Can you work these out from the model? Positions are in its coordinate system, mm. Give positions to 0.01 mm unless a question says otherwise; leave off trailing zeros. Order: outer loops, then holes, each group sorted by start corner. A loop starts at its lowest first (then second) coordinate and runs counter-clockwise, first axis right, second up. Notation, with made-up numbers: M 63,11.5 L 101,11.5 A15 ccw 101,39.5 Z; hole C 82.5,-18 d1. An arc over 180 degrees is marked long. Use one line per item in the form item = value. Start each with the question number.
1. I need wall thicknesses on L1, parallel to X at y = -109, z = 0.95; L2, parallel to Y at x = 61.5, z = 1.2; L3, parallel to Y at x = 182, z = 0.8. Which ranges of each line are inside material? Lowest first, please.
2. I want a section at B-B, the plane x = 152.5. List the corners of the cut face in (y, z) for me.
3. Will these pins go through, and if not, where does the flat tip stop? P1, Ø0.5, axis at x = 234, z = 1.5, coming from the -Y side; P2, Ø0.5, axis at y = -172, z = 1.5, coming from the +X side; P3, Ø0.8, axis at y = -52.5, z = 1.5, coming from the -X side.
4. I want a section at C-C, the plane y = -97. List the corners of the cut face in (x, z) for me, and give its area (3 significant figures).
5. I want a section at A-A, the plane z = 1.55. Count the separate pieces of the cut face and the enclosed holes in it, and give its area (3 significant figures).
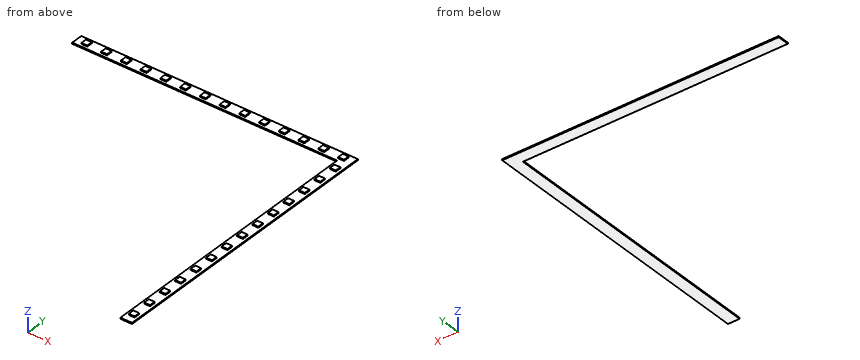
```python
from build123d import *

# Parameters (mm, degrees)
EXTRUDE_1_DEPTH = 1
SKETCH_2_W      = 5
SKETCH_2_H      = 5
EXTRUDE_2_DEPTH = 1


with BuildPart() as part:
    # 草圖1 → 填料-伸長1 (new body)
    with BuildSketch(Plane.XY):
        Polygon((0, 0), (238, 0), (238, -10), (238, -248), (228, -248), (228, -10), (0, -10), align=None)
    extrude(amount=EXTRUDE_1_DEPTH)

    # 草圖2 → 填料-伸長2 (add)
    with BuildSketch(Plane.XY.offset(1)):
        with Locations((25.5, -5)):
            Rectangle(SKETCH_2_W, SKETCH_2_H)
        with Locations((8.5, -5)):
            Rectangle(SKETCH_2_W, SKETCH_2_H)
        with Locations((42.5, -5)):
            Rectangle(SKETCH_2_W, SKETCH_2_H)
        with Locations((59.5, -5)):
            Rectangle(SKETCH_2_W, SKETCH_2_H)
        with Locations((76.5, -5)):
            Rectangle(SKETCH_2_W, SKETCH_2_H)
        with Locations((93.5, -5)):
            Rectangle(SKETCH_2_W, SKETCH_2_H)
        with Locations((110.5, -5)):
            Rectangle(SKETCH_2_W, SKETCH_2_H)
        with Locations((127.5, -5)):
            Rectangle(SKETCH_2_W, SKETCH_2_H)
        with Locations((144.5, -5)):
            Rectangle(SKETCH_2_W, SKETCH_2_H)
        with Locations((161.5, -5)):
            Rectangle(SKETCH_2_W, SKETCH_2_H)
        with Locations((178.5, -5)):
            Rectangle(SKETCH_2_W, SKETCH_2_H)
        with Locations((195.5, -5)):
            Rectangle(SKETCH_2_W, SKETCH_2_H)
        with Locations((212.5, -5)):
            Rectangle(SKETCH_2_W, SKETCH_2_H)
        with Locations((229.5, -5)):
            Rectangle(SKETCH_2_W, SKETCH_2_H)
        with Locations((233, -222.5)):
            Rectangle(SKETCH_2_W, SKETCH_2_H)
        with Locations((233, -239.5)):
            Rectangle(SKETCH_2_W, SKETCH_2_H)
        with Locations((233, -205.5)):
            Rectangle(SKETCH_2_W, SKETCH_2_H)
        with Locations((233, -188.5)):
            Rectangle(SKETCH_2_W, SKETCH_2_H)
        with Locations((233, -171.5)):
            Rectangle(SKETCH_2_W, SKETCH_2_H)
        with Locations((233, -154.5)):
            Rectangle(SKETCH_2_W, SKETCH_2_H)
        with Locations((233, -137.5)):
            Rectangle(SKETCH_2_W, SKETCH_2_H)
        with Locations((233, -120.5)):
            Rectangle(SKETCH_2_W, SKETCH_2_H)
        with Locations((233, -103.5)):
            Rectangle(SKETCH_2_W, SKETCH_2_H)
        with Locations((233, -86.5)):
            Rectangle(SKETCH_2_W, SKETCH_2_H)
        with Locations((233, -69.5)):
            Rectangle(SKETCH_2_W, SKETCH_2_H)
        with Locations((233, -52.5)):
            Rectangle(SKETCH_2_W, SKETCH_2_H)
        with Locations((233, -35.5)):
            Rectangle(SKETCH_2_W, SKETCH_2_H)
        with Locations((233, -18.5)):
            Rectangle(SKETCH_2_W, SKETCH_2_H)
    extrude(amount=EXTRUDE_2_DEPTH)


solid = part.part
```
Check result:
q1.L1 = 228 to 238
q1.L2 = -7.5 to -2.5
q1.L3 = -10 to 0
q2.outline = M -10,0 L 0,0 L 0,1 L -10,1 Z
q3.P1 = -242
q3.P2 = 235.5
q3.P3 = 230.5
q4.outline = M 228,0 L 238,0 L 238,1 L 228,1 Z
q4.area = 10.0 mm2
q5.separate_pieces = 28
q5.enclosed_holes = 0
q5.area = 700 mm2
